Verification items for the finished model (mm, model axes). Face numbers are marked on the shaded views. A direction names the side the tool comes from. Coordinates: 2 decimals unless noted, no trailing zeros. Write each loop counter-clockwise with the first axis right and the second up, starting at its lowest first coordinate (ties: lowest second). Pieces come first, ordered by that corner, then holes. Notation, with made-up numbers: (84.25, 20) -> (132.25, 20) arc R26 ccw to (132.25, 59) -> close; hole circle Ø10 at (75.5, 82). An arc over 180 degrees is marked (long way). Answer in a Markdown table with one row per item.
Autodesk Inventor part; units mm, degrees
ref_plane "YZ Plane" through (0, 0, 0) normal (1, 0, 0) x (0, 1, 0)
ref_plane "XZ Plane" through (0, 0, 0) normal (0, 1, 0) x (-1, 0, 0)
ref_plane "XY Plane" through (0, 0, 0) normal (0, 0, 1) x (1, 0, 0)
sketch "Sketch1" plane through (0, 0, 0) normal (1, 0, 0) x (0, 1, 0)
  line L0 (-4.375, 0) -> (4.375, 0)
  line L1 (4.375, 0) -> (4.375, 10.75)
  line L2 (4.375, 10.75) -> (-4.375, 10.75)
  line L3 (-4.375, 10.75) -> (-4.375, 0)
  circle A0 centre (0, 6.4) radius 3.15
  point P0 (0, 0)
  point P1 (0, 10.75)
  dimension "d0" = 8.75
  dimension "d1" = 10.75
  dimension "d2" = 6.3
  dimension "d3" = 1.2
extrude "Extrusion1" add sketch "Sketch1" along normal blind 3.55
sketch "Sketch2" plane through (0, 0, 0) normal (-1, 0, 0) x (0, 0, 1)
  circle A0 centre (6.4, 0) radius 3.15
  line L0 (0, -4.375) -> (0, 4.375)
  line L1 (10.75, -4.375) -> (0, -4.375)
  line L2 (0, 4.375) -> (10.75, 4.375)
  line L3 (6.3, 4.375) -> (6.3, 3.1484)
  line L4 (6.3, -3.1484) -> (6.3, -4.375)
  point P0 (0, 0)
  dimension "d7" = 6.3
extrude "Extrusion2" add sketch "Sketch2" along normal blind 8.35 contours A0 L4 L1 L0 L2 L3
sketch "Sketch3" plane through (-8.35, 0, 0) normal (-1, 0, 0) x (0, 0, 1)
  line L0 (6.3, -4.375) -> (6.3, -3.1484)
  arc A0 (6.3, 3.1484) -> (6.3, -3.1484) centre (6.4, 0) ccw
  line L1 (6.3, 3.1484) -> (6.3, 4.375)
  arc A1 (6.3, -3.8737) -> (6.3, 3.8737) centre (6.4, 0) ccw
  arc A2 (6.3, -3.1484) -> (6.3, 3.1484) centre (6.4, 0) ccw
  line L2 (6.3, 3.8737) -> (6.3, 3.1484)
  line L3 (6.3, -3.1484) -> (6.3, -3.8737)
  point P0 (0, 0)
  dimension "d10" = 3.875
extrude "Extrusion3" add sketch "Sketch3" against normal up to next contours L0 A2 L1 A1
sketch "Sketch4" plane through (-8.35, 0, 0) normal (-1, 0, 0) x (0, 0, 1)
  circle A0 centre (6.4, 0) radius 3.15
  point P0 (0, 0)
extrude "Extrusion4" add sketch "Sketch4" against normal blind 2.55
sketch "Sketch5" plane through (-8.35, 0, 0) normal (-1, 0, 0) x (0, 0, 1)
  line L0 (6.3, 4.375) -> (0, 4.375)
  line L1 (0, 4.375) -> (0, -4.375)
  line L2 (6.3, -4.375) -> (6.3, -3.8737)
  arc A0 (6.3, -3.8737) -> (6.3, 3.8737) centre (6.4, 0) ccw
  line L3 (7.05, 3.8201) -> (7.05, 2.225)
  line L4 (7.05, 2.225) -> (4.9, 2.225)
  line L5 (4.9, 2.225) -> (4.9, 3.675)
  line L6 (4.9, 3.675) -> (0, 3.675)
  line L7 (6.3, -3.8737) -> (0, -3.8737)
  line L8 (0, 3.675) -> (0, -3.8737)
  arc A1 (6.3, -3.8737) -> (7.05, 3.8201) centre (6.4, 0) ccw
  point P0 (0, 0)
  dimension "d15" = 2.15
  dimension "d17" = 4.9
  dimension "d18" = 0.7
  dimension "d19" = 2.15
extrude "Extrusion5" add sketch "Sketch5" along normal blind 1.6
sketch "Sketch6" plane through (-9.95, 0, 0) normal (-1, 0, 0) x (0, 0, 1)
  line L0 (0, 3.675) -> (0, -3.8737)
  line L1 (0, 3.675) -> (2.8, 3.675)
  line L2 (2.8, 3.675) -> (2.8, 1.4)
  line L3 (2.8, 1.4) -> (0, 1.4)
  line L4 (0, 1.4) -> (0, 3.675)
  line L5 (0, -3.8737) -> (2.8, -3.8737)
  line L6 (2.8, -3.8737) -> (2.8, -1.4)
  line L7 (2.8, -1.4) -> (0, -1.4)
  line L8 (0, -1.4) -> (0, -3.8737)
  arc A0 (6.3, -3.8737) -> (7.05, 3.8201) centre (6.4, 0) ccw
  point P0 (0, 0)
  dimension "d25" = 2.8
  dimension "d28" = 1.4
  dimension "d29" = 1.4
extrude "Extrusion6" add sketch "Sketch6" along normal blind 0.7
equation "\"d29\" = d28"
properties material "ABS Plastic"
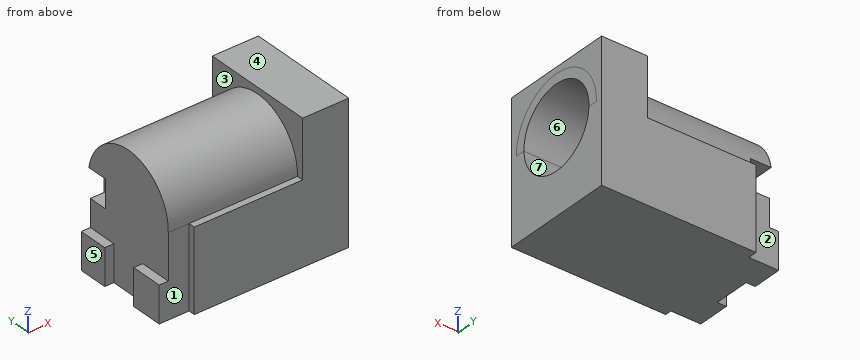
1. Depth check by flat-ended pin: P1, Ø2, axis at x = -2, y = 2, coming from the -Z side; P2, Ø0.6, axis at x = -10, z = 1.5, coming from the +Y side (3 decimals); P3, Ø5, axis at x = -8.5, y = -3.5, coming from the +Z side; P4, Ø1.9, axis at y = -1, z = 8, coming from the +X side. Enter the tip coordinate at first touch or a pass-through.
Geometry says:
| item | result |
|---|---|
| P1 | z = 0 |
| P2 | y = 3.675 |
| P3 | z = 10.14 |
| P4 | x = -5.8 |
2. Thickness scan on line 1 (Y direction, x = -1, z = 6.25) (3 decimals); line 2 (Z direction, x = -1.5, y = 0) (3 decimals); line 3 (Y direction, x = 0.5, z = 8) (3 decimals). Record the ranges inside material, lowest first. Write a range as from..to.
Geometry says:
| item | result |
|---|---|
| line 1 | -4.375..-3.146, 3.146..4.375 |
| line 2 | 0..3.25, 9.55..10.275 |
| line 3 | -4.375..-2.713, 2.713..4.375 |
3. Tool access check on the marked faces 1, 2 and 3. Record the directions out of +Z, -Z, +X, -X, +Y, -Y that give a thin tool (end or side, any length) a straight path to the whole face; none if there is none.
Geometry says:
| item | result |
|---|---|
| face 1 | +Z, -Z, -X, -Y |
| face 2 | -Z, -X, +Y |
| face 3 | +Z, -X |
4. Section check A-A, the plane x = -1.5. Record the boundary of the cut face in (y, z) (3 decimals).
Geometry says:
| item | result |
|---|---|
| outline | (-4.375, 0) -> (4.375, 0) -> (4.375, 6.3) -> (3.874, 6.3) arc R3.875 ccw (long way) to (-3.874, 6.3) -> (-4.375, 6.3) -> close; hole (-3.148, 6.3) arc R3.15 ccw to (3.148, 6.3) arc R3.15 ccw (long way) to start |
5. Section check D-D, the plane x = -7. Record the boundary of the cut face in (y, z) (3 decimals), plus the area to 3 significant figures.
Geometry says:
| item | result |
|---|---|
| outline | (-4.375, 0) -> (4.375, 0) -> (4.375, 6.3) -> (3.874, 6.3) arc R3.875 ccw (long way) to (-3.874, 6.3) -> (-4.375, 6.3) -> close |
| area | 79.5 mm^2 |
6. Mould release check, pull along Z, two halves, no side actions. Record for the marked faces 4, 5, 6 and 7: released by +Z, released by -Z, zero draft, split by the parting line, or undercut.
Geometry says:
| item | result |
|---|---|
| face 4 | released by +Z |
| face 5 | zero draft |
| face 6 | undercut |
| face 7 | undercut |
7. Section check C-C, the plane z = 1.25. Record the boundary of the cut face in (x, y) (3 decimals), plus the area to 3 significant figures.
Geometry says:
| item | result |
|---|---|
| outline | (-10.65, -3.874) -> (-8.35, -3.874) -> (-8.35, -4.375) -> (3.55, -4.375) -> (3.55, 4.375) -> (-8.35, 4.375) -> (-8.35, 3.675) -> (-10.65, 3.675) -> (-10.65, 1.4) -> (-9.95, 1.4) -> (-9.95, -1.4) -> (-10.65, -1.4) -> close |
| area | 120 mm^2 |
8. Section check B-B, the plane y = 0. Record the boundary of the cut face in (x, z) (3 decimals).
Geometry says:
| item | result |
|---|---|
| outline | (-9.95, 0) -> (3.55, 0) -> (3.55, 3.25) -> (-5.8, 3.25) -> (-5.8, 9.55) -> (3.55, 9.55) -> (3.55, 10.75) -> (0, 10.75) -> (0, 10.275) -> (-9.95, 10.275) -> close |
